Verification items for the finished model (mm, model axes). A direction names the side the tool comes from. Coordinates: 2 decimals unless noted, no trailing zeros. Order: outer loops, then holes, each group sorted by start corner. A loop starts at its lowest first (then second) coordinate and runs counter-clockwise, first axis right, second up. Notation, with made-up numbers: M 37.25,20 L 54.25,20 A21 cw 54.25,26 Z; hole C 75,39.25 d8. An arc over 180 degrees is marked long. Return JSON: item names as keys, results as strings. Group by question number.
Q1. Section check C-C, the plane x = 0. Enter the section's corners in (y, z) (3 decimals), then the cut area to 3 significant figures.
Q2. Section check D-D, the plane y = 0.5. Enter the section's corners in (x, z) (3 decimals).
Q3. Thickness scan on probe 1 along X at (y, z) = (-0.55, 0) (3 decimals); probe 2 along X at (y, z) = (1.75, 0.5) (3 decimals); probe 3 along Y at (x, z) = (-3.25, -10). Record the ranges inside material, lowest first.
Q4. Section check B-B, the plane y = 3. Enter the section's corners in (x, z).
Q5. Mould release check, pull along X, two halves, no side actions. Record for faces 1 (the face through (0, 2, 3.5)), 2 (the face through (6, -2.5, -10)), 3 (the face through (14, 1, 0)): pulls with the +X half, pulls with the -X half, needs draft (parallel to the pull), parting line crosses it, or undercut.
Q6. Access from +Z, -Z, +X, -X, +Y, -Y to the whole of each face (thin tool, end or side, straight path). Record for faces 4 (the face through (0, 4.5, 0)), 5 (the face through (-2.5, 3.5, 3)), 6 (the face through (-6.47, -0.04, -8.43)).
Q7. Section check A-A, the plane z = 0. Enter the section's corners in (x, y) (3 decimals), then the cut area to 3 significant figures.
Q8. Go/stop test with a flat-tipped pin: pin 1 Ø5 at (x, z) = (4, 0) entering from -Y. Record where the tip stops, or that it passes through.
from build123d import *

# Parameters (mm, degrees)
SKETCH1_W           = 28
SKETCH1_H           = 28
SKETCH1_R           = 10.625
BOSS_EXTRUDE1_DEPTH = 2.5
SKETCH2_W           = 28
SKETCH2_H           = 28
SKETCH2_W_2         = 1
SKETCH2_H_2         = 6
BOSS_EXTRUDE2_DEPTH = 2
BOSS_EXTRUDE3_DEPTH = 3
CHAMFER1_SIZE       = 1


with BuildPart() as part:
    # Sketch1 → Boss-Extrude1 (new, symmetric)
    with BuildSketch(Plane(origin=(0, 0, 0), x_dir=(1, 0, 0), z_dir=(0, 1, 0))):
        Rectangle(SKETCH1_W, SKETCH1_H)
        with Locations(Location((0, 0, 0), (0, 0, 270))):
            Circle(SKETCH1_R, mode=Mode.SUBTRACT)
    extrude(amount=BOSS_EXTRUDE1_DEPTH, both=True)

    # Sketch2 → Boss-Extrude2 (add)
    with BuildSketch(Plane(origin=(0, 2.5, 0), x_dir=(1, 0, 0), z_dir=(0, 1, 0))):
        Rectangle(SKETCH2_W, SKETCH2_H)
        with Locations((-2.5, 0)):
            Rectangle(SKETCH2_W_2, SKETCH2_H_2, mode=Mode.SUBTRACT)
        with Locations((2.5, 0)):
            Rectangle(SKETCH2_W_2, SKETCH2_H_2, mode=Mode.SUBTRACT)
    extrude(amount=BOSS_EXTRUDE2_DEPTH)

    # Sketch3 → Boss-Extrude3 (add, symmetric)
    with BuildSketch(Plane.XY):
        with BuildLine():
            Line((-2, 2.5), (2, 2.5))
            ThreePointArc((2, 2.5), (0, 0.97783361), (-2, 2.5))
        make_face()
    extrude(amount=BOSS_EXTRUDE3_DEPTH, both=True)

    # Chamfer1
    # the kernel refuses this chamfer: 1 mm, written as the material it adds along each edge
    with BuildSketch(Plane(origin=(-4.571682988, 2.5, -3), x_dir=(0, 0.027495876610586487, -0.9996219169112968), z_dir=(1, 0, 0))) as chamfer1_piece_1_section:
        Polygon((CHAMFER1_SIZE * 0.999621916911, -CHAMFER1_SIZE * 0.0274958766106), (-CHAMFER1_SIZE * 0.0274958766106, -CHAMFER1_SIZE * 0.999621916911), (0, 0), align=None)
    chamfer1_piece_1 = extrude(amount=9.143365976, mode=Mode.PRIVATE)
    chamfer1_piece_1 = chamfer1_piece_1 & Plane(origin=(0, 3.05283361, -3.341258545), x_dir=(0.9638554216867474, -0.266425835993926, 0), z_dir=(0, 0, 1)) * Cylinder(2.075, 23, mode=Mode.PRIVATE)
    add(chamfer1_piece_1)
    with BuildSketch(Plane(origin=(-4.571682988, 2.5, 3), x_dir=(0, 0.027495876610586487, 0.9996219169112968), z_dir=(1, 0, 0))) as chamfer1_piece_2_section:
        Polygon((CHAMFER1_SIZE * 0.999621916911, CHAMFER1_SIZE * 0.0274958766106), (-CHAMFER1_SIZE * 0.0274958766106, CHAMFER1_SIZE * 0.999621916911), (0, 0), align=None)
    chamfer1_piece_2 = extrude(amount=9.143365976, mode=Mode.PRIVATE)
    chamfer1_piece_2 = chamfer1_piece_2 & Plane(origin=(0, 3.05283361, 3.341258545), x_dir=(0.9638554216867474, -0.266425835993926, 0), z_dir=(0, 0, 1)) * Cylinder(2.075, 23, mode=Mode.PRIVATE)
    add(chamfer1_piece_2)


solid = part.part
Numbers:
{
 "1": {"outline": "M -2.5,-14 L 4.5,-14 L 4.5,14 L -2.5,14 L -2.5,10.625 L 2.5,10.625 L 2.5,4 L 1.5,3 L 0.978,3 L 0.978,-3 L 1.5,-3 L 2.5,-4 L 2.5,-10.625 L -2.5,-10.625 Z", "area": "99.9 mm2"},
 "2": {"outline": "M -14,-14 L 14,-14 L 14,14 L -14,14 Z; hole C 0,0 d21.25"},
 "3": {"probe 1": "x = -14 to -10.625, 10.625 to 14", "probe 2": "x = -14 to -10.613, -1.615 to 1.615, 10.613 to 14", "probe 3": "y = 2.5 to 4.5"},
 "4": {"outline": "M -14,-14 L 14,-14 L 14,14 L -14,14 Z; hole M -3,-3 L -2,-3 L -2,3 L -3,3 Z; hole M 2,-3 L 3,-3 L 3,3 L 2,3 Z"},
 "5": {"face 1": "undercut", "face 2": "needs draft", "face 3": "pulls with the +X half"},
 "6": {"face 4": "+Z, -Z, +X, -X, +Y", "face 5": "+Y, -Y", "face 6": "-Y"},
 "7": {"outline": "M -14,-2.5 L -10.625,-2.5 L -10.625,2.5 L -3,2.5 L -3,4.5 L -14,4.5 Z; M -2,2.5 A2.075 ccw 2,2.5 L 2,4.5 L -2,4.5 Z; M 3,2.5 L 10.625,2.5 L 10.625,-2.5 L 14,-2.5 L 14,4.5 L 3,4.5 Z", "area": "90.2 mm2"},
 "8": {"pin 1": "stops at y = 1.62"}
}
